Check sheet for the modelled part. Datum: model origin and axes. Units: mm. Give positions to 0.01 mm unless a question says otherwise; leave off trailing zeros. Write each loop counter-clockwise with the first axis right and the second up, starting at its lowest first coordinate (ties: lowest second). Pieces come first, ordered by that corner, then holes.
from build123d import *

# Parameters (mm, degrees)
F0_R          = 8
F0_W          = 1.75
F0_H          = 1.75
F0_R_2        = 0.85
F1_DEPTH      = 0.75
F1_DEPTH_BACK = 0.75
F2_R          = 0.6


with BuildPart() as f1:
    # F0 (on Top) → F1 (new body, two sides)
    with BuildSketch(Plane.XY) as f1_sk:
        Circle(F0_R)
        with BuildLine():
            ThreePointArc((0.875, 6.440836514), (4.5961940777, 4.5961940777), (6.440836514, 0.875))
            Line((6.440836514, 0.875), (7.3671648279, 0.875))
            Line((7.3671648279, 0.875), (7.3671648279, -0.875))
            Line((7.3671648279, -0.875), (6.440836514, -0.875))
            ThreePointArc((6.440836514, -0.875), (4.5961940777, -4.5961940777), (0.875, -6.440836514))
            Line((0.875, -6.440836514), (0.875, -6.9778915495))
            Line((0.875, -6.9778915495), (-0.875, -6.9778915495))
            Line((-0.875, -6.9778915495), (-0.875, -6.440836514))
            ThreePointArc((-0.875, -6.440836514), (-4.5961940777, -4.5961940777), (-6.440836514, -0.875))
            Line((-6.440836514, -0.875), (-7.3671648279, -0.875))
            Line((-7.3671648279, -0.875), (-7.3671648279, 0.875))
            Line((-7.3671648279, 0.875), (-6.440836514, 0.875))
            ThreePointArc((-6.440836514, 0.875), (-4.5961940777, 4.5961940777), (-0.875, 6.440836514))
            Line((-0.875, 6.440836514), (-0.875, 6.9778915495))
            Line((-0.875, 6.9778915495), (0.875, 6.9778915495))
            Line((0.875, 6.9778915495), (0.875, 6.440836514))
        make_face(mode=Mode.SUBTRACT)
        with BuildLine():
            Line((-1.7984368212, 0.875), (-6.440836514, 0.875))
            ThreePointArc((-6.440836514, 0.875), (-6.5, 0), (-6.440836514, -0.875))
            Line((-6.440836514, -0.875), (-1.7984368212, -0.875))
            ThreePointArc((-1.7984368212, -0.875), (-2, 0), (-1.7984368212, 0.875))
        make_face()
        with BuildLine():
            Line((0.875, 1.7984368212), (0.875, 6.440836514))
            ThreePointArc((0.875, 6.440836514), (0, 6.5), (-0.875, 6.440836514))
            Line((-0.875, 6.440836514), (-0.875, 1.7984368212))
            ThreePointArc((-0.875, 1.7984368212), (0, 2), (0.875, 1.7984368212))
        make_face()
        with BuildLine():
            ThreePointArc((6.440836514, -0.875), (6.4851922616, -0.4384989504), (6.5, 0))
            ThreePointArc((6.5, 0), (6.4851922616, 0.4384989504), (6.440836514, 0.875))
            Line((6.440836514, 0.875), (1.7984368212, 0.875))
            ThreePointArc((1.7984368212, 0.875), (1.9489578808, 0.4489578808), (2, 0))
            ThreePointArc((2, 0), (1.9489578808, -0.4489578808), (1.7984368212, -0.875))
            Line((1.7984368212, -0.875), (6.440836514, -0.875))
        make_face()
        with BuildLine():
            ThreePointArc((-0.875, -6.440836514), (0, -6.5), (0.875, -6.440836514))
            Line((0.875, -6.440836514), (0.875, -1.7984368212))
            ThreePointArc((0.875, -1.7984368212), (0, -2), (-0.875, -1.7984368212))
            Line((-0.875, -1.7984368212), (-0.875, -6.440836514))
        make_face()
        Rectangle(F0_W, F0_H)
        Circle(F0_R_2, mode=Mode.SUBTRACT)
        with BuildLine():
            Line((0.875, 0.875), (0.875, 1.7984368212))
            ThreePointArc((0.875, 1.7984368212), (0, 2), (-0.875, 1.7984368212))
            Line((-0.875, 1.7984368212), (-0.875, 0.875))
            Line((-0.875, 0.875), (0.875, 0.875))
        make_face()
        with BuildLine():
            Line((-0.875, -0.875), (-0.875, 0.875))
            Line((-0.875, 0.875), (-1.7984368212, 0.875))
            ThreePointArc((-1.7984368212, 0.875), (-2, 0), (-1.7984368212, -0.875))
            Line((-1.7984368212, -0.875), (-0.875, -0.875))
        make_face()
        with BuildLine():
            ThreePointArc((-0.875, -1.7984368212), (0, -2), (0.875, -1.7984368212))
            Line((0.875, -1.7984368212), (0.875, -0.875))
            Line((0.875, -0.875), (-0.875, -0.875))
            Line((-0.875, -0.875), (-0.875, -1.7984368212))
        make_face()
        with BuildLine():
            ThreePointArc((2, 0), (1.9489578808, 0.4489578808), (1.7984368212, 0.875))
            Line((1.7984368212, 0.875), (0.875, 0.875))
            Line((0.875, 0.875), (0.875, -0.875))
            Line((0.875, -0.875), (1.7984368212, -0.875))
            ThreePointArc((1.7984368212, -0.875), (1.9489578808, -0.4489578808), (2, 0))
        make_face()
        with BuildLine():
            ThreePointArc((-6.440836514, -0.875), (-6.5, 0), (-6.440836514, 0.875))
            Line((-6.440836514, 0.875), (-7.3671648279, 0.875))
            Line((-7.3671648279, 0.875), (-7.3671648279, -0.875))
            Line((-7.3671648279, -0.875), (-6.440836514, -0.875))
        make_face()
        with BuildLine():
            ThreePointArc((6.440836514, 0.875), (6.4851922616, 0.4384989504), (6.5, 0))
            ThreePointArc((6.5, 0), (6.4851922616, -0.4384989504), (6.440836514, -0.875))
            Line((6.440836514, -0.875), (7.3671648279, -0.875))
            Line((7.3671648279, -0.875), (7.3671648279, 0.875))
            Line((7.3671648279, 0.875), (6.440836514, 0.875))
        make_face()
        with BuildLine():
            ThreePointArc((-0.875, 6.440836514), (0, 6.5), (0.875, 6.440836514))
            Line((0.875, 6.440836514), (0.875, 6.9778915495))
            Line((0.875, 6.9778915495), (-0.875, 6.9778915495))
            Line((-0.875, 6.9778915495), (-0.875, 6.440836514))
        make_face()
        with BuildLine():
            Line((0.875, -6.9778915495), (0.875, -6.440836514))
            ThreePointArc((0.875, -6.440836514), (0, -6.5), (-0.875, -6.440836514))
            Line((-0.875, -6.440836514), (-0.875, -6.9778915495))
            Line((-0.875, -6.9778915495), (0.875, -6.9778915495))
        make_face()
        with BuildLine():
            Line((0.875, 0.875), (1.7984368212, 0.875))
            ThreePointArc((1.7984368212, 0.875), (1.4142135624, 1.4142135624), (0.875, 1.7984368212))
            Line((0.875, 1.7984368212), (0.875, 0.875))
        make_face()
        with BuildLine():
            Line((-0.875, 0.875), (-0.875, 1.7984368212))
            ThreePointArc((-0.875, 1.7984368212), (-1.4142135624, 1.4142135624), (-1.7984368212, 0.875))
            Line((-1.7984368212, 0.875), (-0.875, 0.875))
        make_face()
        with BuildLine():
            ThreePointArc((-1.7984368212, -0.875), (-1.4142135624, -1.4142135624), (-0.875, -1.7984368212))
            Line((-0.875, -1.7984368212), (-0.875, -0.875))
            Line((-0.875, -0.875), (-1.7984368212, -0.875))
        make_face()
        with BuildLine():
            ThreePointArc((0.875, -1.7984368212), (1.4142135624, -1.4142135624), (1.7984368212, -0.875))
            Line((1.7984368212, -0.875), (0.875, -0.875))
            Line((0.875, -0.875), (0.875, -1.7984368212))
        make_face()
    extrude(amount=F1_DEPTH)
    extrude(f1_sk.sketch, amount=-F1_DEPTH_BACK)

    # F2
    f2_edges = [f1.edges().sort_by_distance(p)[0] for p in [
        (-8, 0, 0.75),
        (-4.596194, -4.596194, 0.75),
        (-4.119637, -0.875, 0.75),
        (-4.119637, 0.875, 0.75),
        (-0.875, 4.119637, 0.75),
        (0.875, 4.119637, 0.75),
        (-4.596194, 4.596194, 0.75),
        (4.596194, 4.596194, 0.75),
        (4.119637, 0.875, 0.75),
        (4.119637, -0.875, 0.75),
        (4.596194, -4.596194, 0.75),
        (0.875, -4.119637, 0.75),
        (-0.875, -4.119637, 0.75),
        (-8, 0, -0.75),
        (4.596194, -4.596194, -0.75),
        (4.119637, -0.875, -0.75),
        (0.875, -4.119637, -0.75),
        (-0.875, -4.119637, -0.75),
        (-4.596194, -4.596194, -0.75),
        (-4.119637, -0.875, -0.75),
        (-4.119637, 0.875, -0.75),
        (-4.596194, 4.596194, -0.75),
        (4.596194, 4.596194, -0.75),
        (4.119637, 0.875, -0.75),
        (-0.875, 4.119637, -0.75),
        (0.875, 4.119637, -0.75),
    ]]
    fillet(f2_edges, radius=F2_R)


solid = f1.part
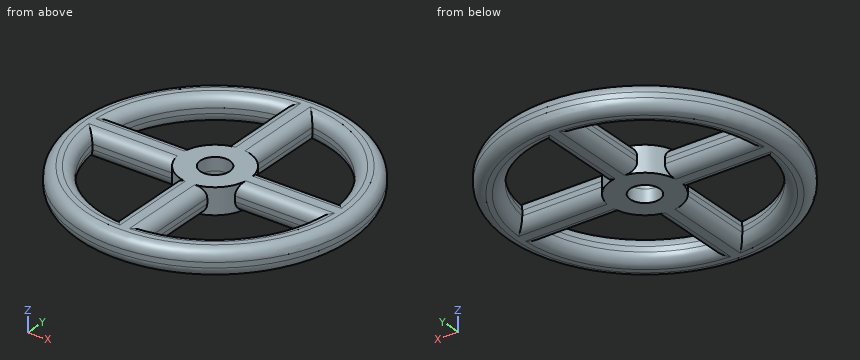
1) Sectioned sample at D-D on y = -3.5. Give the number of separate pieces and of enclosed holes in the cut face, then the cut area to 3 significant figures.
2) Sectioned sample at A-A on y = 0. Record the boundary of the cut face in (x, z), then the cut area to 3 significant figures.
3) Gauge pin test, flat end, axial feed: pin 1 (8 mm diameter, centred on x = 3.5, y = 5.5, fed in from +Z). Record the tip position at first contact, or that the pin passes through.
4) Scan lines: L1, parallel to X at y = 4.25, z = 0.5; L2, parallel to X at y = 3.75, z = 0.1 (3 decimals); L3, parallel to Y at x = 3.5, z = -0.55. Record each from-to range of solid material in increasing order.
5) Sectioned sample at C-C on z = -0.45. Record the boundary of the cut face in (x, y), then the cut area to 3 significant figures.
Answers below:
1. separate pieces: 3
1. enclosed holes: 0
1. area: 6.76 mm2
2. outline: (-8, -0.15) arc R0.6 ccw to (-7.4, -0.75) - (-0.85, -0.75) - (-0.85, 0.75) - (-7.4, 0.75) arc R0.6 ccw to (-8, 0.15) - close; (0.85, -0.75) - (7.4, -0.75) arc R0.6 ccw to (8, -0.15) - (8, 0.15) arc R0.6 ccw to (7.4, 0.75) - (0.85, 0.75) - close
2. area: 21.1 mm2
3. pin 1: stops at z = 0.75
4. L1: x = -6.64 to -5.07, -0.76 to 0.76, 5.07 to 6.64
4. L2: x = -7.067 to -5.309, -0.875 to 0.875, 5.309 to 7.067
4. L3: y = -7.02 to -5.66, -0.72 to 0.72, 5.66 to 7.02
5. outline: circle Ø15.84 at (0, 0); hole (-6.53, -0.79) arc R6.58 ccw to (-0.79, -6.53) - (-0.79, -1.84) arc R2 cw to (-1.84, -0.79) - close; hole (-6.53, 0.79) - (-1.84, 0.79) arc R2 cw to (-0.79, 1.84) - (-0.79, 6.53) arc R6.58 ccw to start; hole circle Ø1.7 at (0, 0); hole (0.79, -6.53) arc R6.58 ccw to (6.53, -0.79) - (1.84, -0.79) arc R2 cw to (0.79, -1.84) - close; hole (0.79, 1.84) arc R2 cw to (1.84, 0.79) - (6.53, 0.79) arc R6.58 ccw to (0.79, 6.53) - close
5. area: 101 mm2
